from build123d import *

# Parameters (mm, degrees)
SKETCH1_W               = 25.4
SKETCH1_H               = 50.8
SKETCH1_W_2             = 19.05
SKETCH1_H_2             = 44.45
BOSS_EXTRUDE1_DEPTH     = 304.8
F_10_CLEARANCE_HOLE1_D  = 5.1054
F_1_4_CLEARANCE_HOLE2_D = 6.7564
SKETCH7_R               = 14.2875
SKETCH7_R_2             = 3.175
CUT_EXTRUDE1_DEPTH      = 307.909367729
SKETCH8_R               = 2.5527
CUT_EXTRUDE2_DEPTH      = 307.909367729


with BuildPart() as part:
    # Sketch1 → Boss-Extrude1 (new, symmetric)
    with BuildSketch(Plane.XY):
        Rectangle(SKETCH1_W, SKETCH1_H)
        Rectangle(SKETCH1_W_2, SKETCH1_H_2, mode=Mode.SUBTRACT)
    extrude(amount=BOSS_EXTRUDE1_DEPTH, both=True)

    # #10 Clearance Hole1 (through all)
    with Locations(Plane(origin=(12.7, 0, 0), x_dir=(0, 0, -1), z_dir=(1, 0, 0))):
        with Locations((-292.1, 12.7), (-292.1, 0), (-292.1, -12.7)):
            f_10_clearance_hole1 = Hole(F_10_CLEARANCE_HOLE1_D / 2)

    # Mirror1: #10 Clearance Hole1 across plane
    add(f_10_clearance_hole1.mirror(Plane.XY), mode=Mode.SUBTRACT)

    # 1/4 Clearance Hole2 (through all)
    with Locations(Plane(origin=(12.7, 0, 0), x_dir=(0, 0, -1), z_dir=(1, 0, 0))):
        with Locations((-38.1, 0), (38.1, 0), (-104.14, 0), (104.14, 0)):
            Hole(F_1_4_CLEARANCE_HOLE2_D / 2)

    # Sketch7 → Cut-Extrude1 (cut, through all)
    with BuildSketch(Plane(origin=(12.7, 0, 0), x_dir=(0, 0, -1), z_dir=(1, 0, 0))):
        with Locations(Location((-228.6762, 0, 0), (0, 0, 90))):
            Circle(SKETCH7_R)
        with Locations(Location((177.7238, 0, 0), (0, 0, 90))):
            Circle(SKETCH7_R)
        with Locations(Location((228.6, 0, 0), (0, 0, 90))):
            Circle(SKETCH7_R)
        with Locations(Location((139.6238, 0, 0), (0, 0, 90))):
            Circle(SKETCH7_R_2)
        with Locations(Location((266.7, 0, 0), (0, 0, 90))):
            Circle(SKETCH7_R_2)
    extrude(amount=-CUT_EXTRUDE1_DEPTH, mode=Mode.SUBTRACT)

    # Sketch8 → Cut-Extrude2 (cut, through all)
    with BuildSketch(Plane(origin=(12.7, 0, 0), x_dir=(0, 0, -1), z_dir=(1, 0, 0))):
        with Locations(Location((140.97, 12.7, 0), (0, 0, 90))):
            Circle(SKETCH8_R)
        with Locations(Location((140.97, -12.7, 0), (0, 0, 90))):
            Circle(SKETCH8_R)
    extrude(amount=-CUT_EXTRUDE2_DEPTH, mode=Mode.SUBTRACT)


solid = part.part
The model under review builds one solid part; all positions refer to its coordinate system, in mm. A direction names the side the tool comes from. Give positions to 0.01 mm unless a question says otherwise; leave off trailing zeros. Loops run counter-clockwise (first coordinate to the right, second up) from the corner with the lowest first, then second, coordinate; pieces in that order, holes last. Notation, with made-up numbers: (7, 2) -> (38, 2) arc R16 ccw to (38, 11) -> close; hole circle Ø3 at (46.25, 69). An arc over 180 degrees is marked (long way). Answer as a JSON object with one key per item and string values. Group by question number.
Q1. Draft analysis for pull direction Y (two halves, no side actions). For faces 1 (the cylindrical face through (-11.09, -3.1, -191.67)), 2 (the cylindrical face through (-11.09, -3.1, 214.73)), 3 (the flat face through (-12.7, 0, 4)), 4 (the flat face through (0, 25.4, 4)), state which applies: pulls with the +Y half, pulls with the -Y half, needs draft (parallel to the pull), parting line crosses it, or undercut.
Q2. Insertion check: pin 1 (3 mm diameter, centred on y = -12.7, z = -140.97, fed in from +X); pin 2 (10 mm diameter, centred on y = 0, z = -139.62, fed in from -X). Each pin has a flat end and moves straight along its axis. Give the tip position at first contact, or say it passes through.
Q3. Take a section at B-B (x = 5.5). Write out the cut boundary in (y, z) (3 decimals), plus the area to 3 significant figures.
Q4. Wall thickness on line 1 along Y through (x, z) = (-11.6, -292.1); line 2 along Y through (x, z) = (5.75, 35) (3 decimals); line 3 along X through (y, z) = (-16.5, 81) (3 decimals): over which ranges is each line inside the solid? List them lowest first.
Q5. Tool access review of faces 5 (the flat face through (0, -22.225, 4)), 6 (the flat face through (-10, -2, 304.8)): name each direction out of +Z, -Z, +X, -X, +Y, -Y from which nothing blocks a thin tool from reaching the whole face with its end or side.
Q6. Take a section at A-A (z = 155.5). Write out the cut boundary in (x, y) (3 decimals), plus the area to 3 significant figures.
Answer below:
{
 "1": {"face 1": "undercut", "face 2": "undercut", "face 3": "needs draft", "face 4": "pulls with the +Y half"},
 "2": {"pin 1": "passes through", "pin 2": "stops at x = -12.7"},
 "3": {"outline": "(-25.4, -304.8) -> (-22.225, -304.8) -> (-22.225, 304.8) -> (-25.4, 304.8) -> close; (22.225, -304.8) -> (25.4, -304.8) -> (25.4, 304.8) -> (22.225, 304.8) -> close", "area": "3,870 mm2"},
 "4": {"line 1": "y = -25.4 to -15.25, -10.15 to -2.55, 2.55 to 10.15, 15.25 to 25.4", "line 2": "y = -25.4 to -22.225, 22.225 to 25.4", "line 3": "x = -12.7 to -9.525, 9.525 to 12.7"},
 "5": {"face 5": "+Z, -Z", "face 6": "+Z, +X, -X, +Y, -Y"},
 "6": {"outline": "(-12.7, -25.4) -> (12.7, -25.4) -> (12.7, 25.4) -> (-12.7, 25.4) -> close; hole (-9.525, -22.225) -> (9.525, -22.225) -> (9.525, 22.225) -> (-9.525, 22.225) -> close", "area": "444 mm2"}
}
